Build history of the part. All positions in model axes, mm. Face numbers are marked on the shaded views. A direction names the side the tool comes from. Round coordinates to 2 decimals unless told otherwise and drop trailing zeros. Write each loop counter-clockwise with the first axis right and the second up, starting at its lowest first coordinate (ties: lowest second). Pieces come first, ordered by that corner, then holes. Notation, with made-up numbers: M 16,3 L 41,3 A20 cw 41,42 Z; hole C 76,59.5 d4. An arc over 180 degrees is marked long. Write item = value, one per line.
from build123d import *

# Parameters (mm, degrees)
SKETCH1_W           = 30
SKETCH1_H           = 20
BOSS_EXTRUDE1_DEPTH = 30


with BuildPart() as part:
    # Sketch1 → Boss-Extrude1 (new, symmetric)
    with BuildSketch(Plane.XY):
        Polygon((33.229508197, -36.442622951), (-46.770491803, -36.442622951), (-46.770491803, -26.442622951), (-31.770491803, -26.442622951), (-31.770491803, 3.557377049), (-46.770491803, 3.557377049), (-46.770491803, 13.557377049), (33.229508197, 13.557377049), (33.229508197, 3.557377049), (18.229508197, 3.557377049), (18.229508197, -26.442622951), (33.229508197, -26.442622951), align=None)
        with Locations((-6.770491803, -11.442622951)):
            Rectangle(SKETCH1_W, SKETCH1_H, mode=Mode.SUBTRACT)
    extrude(amount=BOSS_EXTRUDE1_DEPTH, both=True)


solid = part.part
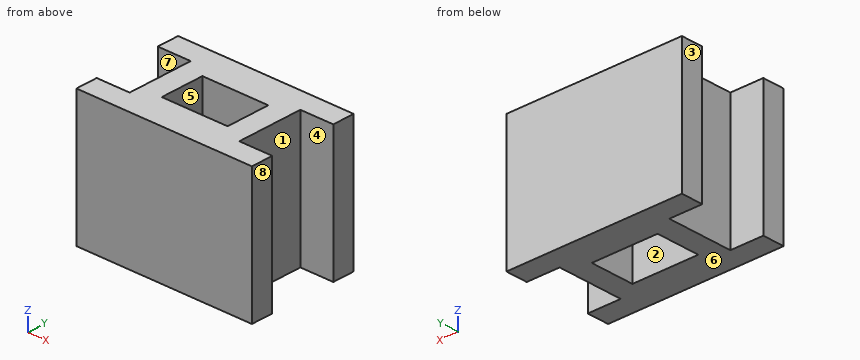
1. Band-saw the part on C-C (y = -19.5). List the corners of the cut face in (x, z).
Responses:
outline = M -31.77,-30 L -21.77,-30 L -21.77,30 L -31.77,30 Z; M 8.23,-30 L 18.23,-30 L 18.23,30 L 8.23,30 Z
2. Band-saw the part on D-D (y = -25). List the corners of the cut face in (x, z), plus the area to 3 significant figures.
Responses:
outline = M -31.77,-30 L 18.23,-30 L 18.23,30 L -31.77,30 Z
area = 3,000 mm²
3. Band-saw the part on A-A (x = 6). List the corners of the cut face in (y, z), plus the area to 3 significant figures.
Responses:
outline = M -36.44,-30 L -21.44,-30 L -21.44,30 L -36.44,30 Z; M -1.44,-30 L 13.56,-30 L 13.56,30 L -1.44,30 Z
area = 1,800 mm²
4. Band-saw the part on B-B (z = -5). List the corners of the cut face in (x, y).
Responses:
outline = M -46.77,-36.44 L 33.23,-36.44 L 33.23,-26.44 L 18.23,-26.44 L 18.23,3.56 L 33.23,3.56 L 33.23,13.56 L -46.77,13.56 L -46.77,3.56 L -31.77,3.56 L -31.77,-26.44 L -46.77,-26.44 Z; hole M -21.77,-21.44 L 8.23,-21.44 L 8.23,-1.44 L -21.77,-1.44 Z
5. Mould opens along X. For the marked faces 1, 2 and 3 say: pulls with the +X half, pulls with the -X half, needs draft (parallel to the pull), parting line crosses it, or undercut.
Responses:
face_1 = pulls with the +X half
face_2 = undercut
face_3 = pulls with the -X half
6. Flat gauge pins, fed straight in: pin 1 (6 mm diameter, centred on y = -12.5, z = -3.5, fed in from -X); pin 2 (6 mm diameter, centred on y = -14.5, z = -14, fed in from +X). Where does each tip first touch, or does it go through?
Responses:
pin_1 = -31.77
pin_2 = 18.23
7. Probe probe 1 along Y at (x, z) = (18.5, -18.5); probe 2 along X at (y, z) = (-8.5, 6.5); probe 3 along Y at (x, z) = (-10.5, -11). List the from-to ranges inside material, lowest first.
Responses:
probe_1 = -36.44 to -26.44, 3.56 to 13.56
probe_2 = -31.77 to -21.77, 8.23 to 18.23
probe_3 = -36.44 to -21.44, -1.44 to 13.56
8. Tool access for the marked faces 4, 5, 6, 7 and 8: list every direction of +Z, -Z, +X, -X, +Y, -Y with a clear straight run to the whole face (end or side of a thin tool).
Responses:
face_4 = +Z, -Z, +X
face_5 = +Z, -Z
face_6 = -Z, +X, -X, +Y, -Y
face_7 = +Z, -Z, -X
face_8 = +Z, -Z, +X, +Y, -Y
